Here's the drawing with two shaded views (mm, measured from the low corner). I have some questions. A direction names the side the tool comes from. Round coordinates to 2 decimals unless told otherwise and drop trailing zeros. Order: outer loops, then holes, each group sorted by start corner. A loop starts at its lowest first (then second) coordinate and runs counter-clockwise, first axis right, second up.
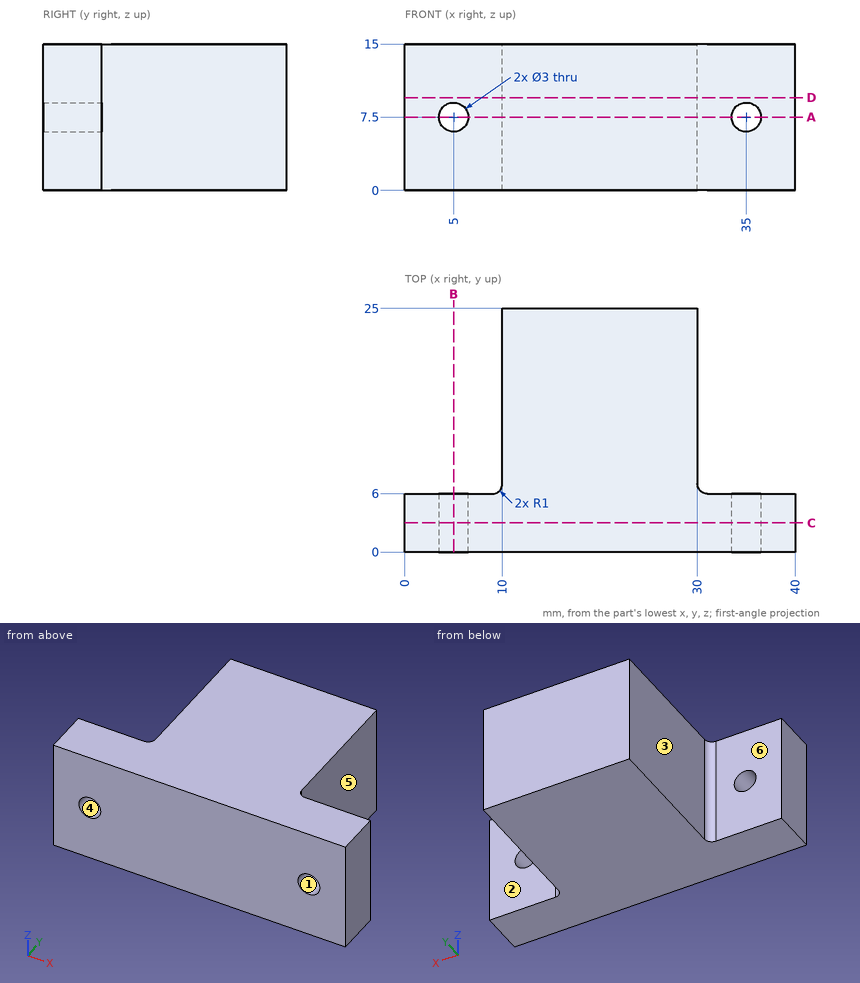
1. If we section it at B-B, the plane x = 5: Write out the boundary of the cut face in (y, z), and give its area (3 significant figures).
Evaluation:
outline: (0, 0) - (6, 0) - (6, 6) - (0, 6) - close; (0, 9) - (6, 9) - (6, 15) - (0, 15) - close
area: 72.0 mm2
2. If we section it at D-D, the plane z = 9.5: Write out the boundary of the cut face in (x, y), and give its area (3 significant figures).
Evaluation:
outline: (0, 0) - (40, 0) - (40, 6) - (31, 6) arc R1 cw to (30, 7) - (30, 25) - (10, 25) - (10, 7) arc R1 cw to (9, 6) - (0, 6) - close
area: 620 mm2
3. If we mould it in two halves opening along X, with no side actions, what happens to the marked faces 4, 5 and 6? For each: released by +X, released by -X, zero draft, split by the parting line, or undercut.
Evaluation:
face 4: undercut
face 5: released by +X
face 6: zero draft
4. If we section it at C-C, the plane y = 3: Write out the boundary of the cut face in (x, z), and give its area (3 significant figures).
Evaluation:
outline: (0, 0) - (40, 0) - (40, 15) - (0, 15) - close; hole circle Ø3 at (5, 7.5); hole circle Ø3 at (35, 7.5)
area: 586 mm2
5. If we section it at A-A, the plane z = 7.5: Write out the boundary of the cut face in (x, y), and give its area (3 significant figures).
Evaluation:
outline: (0, 0) - (3.5, 0) - (3.5, 6) - (0, 6) - close; (6.5, 0) - (33.5, 0) - (33.5, 6) - (31, 6) arc R1 cw to (30, 7) - (30, 25) - (10, 25) - (10, 7) arc R1 cw to (9, 6) - (6.5, 6) - close; (36.5, 0) - (40, 0) - (40, 6) - (36.5, 6) - close
area: 584 mm2
6. On a 3-axis mill with a long thin cutter (end or side, diameter ignored), from which of +Z, -Z, +X, -X, +Y, -Y can I reach the whole of each face in a straight line? I mean the marked faces 1, 2 and 3. Say none if no direction works.
Evaluation:
face 1: +Y, -Y
face 2: +Z, -Z, +X, +Y
face 3: +Z, -Z, -X, +Y
7. I'm going to push flat-ended pins straight in: P1, Ø2, axis at x = 33.5, z = 4.5, coming from the +Y side; P2, Ø8, axis at y = 20.5, z = 7.5, coming from the -X side; P3, Ø8, axis at x = 7, z = 12.5, coming from the +Y side. Where does each tip first touch, or does it pass through?
Evaluation:
P1: stops at y = 6
P2: stops at x = 10
P3: stops at y = 25
8. I need wall thicknesses on probe 1 along Z at (x, y) = (5, 3.4); probe 2 along Y at (x, z) = (6, 5.5); probe 3 along X at (y, z) = (18.75, 2). Which ranges of each line are inside material? Lowest first, please.
Evaluation:
probe 1: z = 0 to 6, 9 to 15
probe 2: y = 0 to 6
probe 3: x = 10 to 30
